Could you check a few things on this model? Use its own coordinates, in mm. Round coordinates to 2 decimals unless told otherwise and drop trailing zeros. Loops run counter-clockwise (first coordinate to the right, second up) from the corner with the lowest first, then second, coordinate; pieces in that order, holes last. Notation, with made-up numbers: (-27.5, -30.75) -> (-12.5, -30.75) arc R31 cw to (-12.5, 4.25) -> close; hole circle Ø10 at (62.5, 13.5). An arc over 180 degrees is marked (long way). Write each question's results on one line, items separated by ' | '. Start each with the question number.
1) For P1, Ø1, axis at y = -4, z = 2, coming from the -X side; P2, Ø2, axis at x = 141, z = 2, coming from the -Y side, each with a flat end and sliding along its axis, tell me the tip position at first contact or that it passes through.
2) Imagine slicing it at A-A, the plane z = 1. Give the number of separate pieces and of enclosed holes in the cut face, plus the area to 3 significant figures.
3) If I drill on probe 1 along X at (y, z) = (-7.5, 4.75); probe 2 along Y at (x, z) = (153, 2.75); probe 3 along X at (y, z) = (-2, 1.75), over which ranges is the centre line in solid material (lowest first)?
4) Imagine slicing it at C-C, the plane y = -27. List the corners of the cut face in (x, z) for me, plus the area to 3 significant figures.
5) Imagine slicing it at B-B, the plane x = 162.5. List the corners of the cut face in (y, z) for me, plus the area to 3 significant figures.
from build123d import *

# Parameters (mm, degrees)
BOSS_EXTRUDE1_DEPTH       = 6.604
F_6_CLEARANCE_HOLE1_D     = 3.6576
F_6_CLEARANCE_HOLE1_DEPTH = 10.16
F_6_CLEARANCE_HOLE1_TIP   = 1.0988539


with BuildPart() as part:
    # Sketch1 → Boss-Extrude1 (new body)
    with BuildSketch(Plane.XY):
        with BuildLine():
            Line((16.823092539, -23.059379431), (270.045750863, -45.152940848))
            Line((270.045750863, -45.152940848), (271.149626418, -32.501005867))
            Line((271.149626418, -32.501005867), (18.308001968, -10.440689482))
            add(Edge.make_bspline(
                [(6.100873241, 1.761205752), (6.243998722, 1.265414493), (6.562029623, 0.258197332), (7.239782187, -1.541714319), (8.191856686, -3.521031278), (9.459597024, -5.451591955), (10.839105985, -7.00109828), (12.345816988, -8.235279198), (14.031634784, -9.215214087), (15.656369367, -9.844087266), (17.105920915, -10.226590441), (17.911821211, -10.379141677), (18.308001968, -10.440689482)],
                knots=[0, 0, 0, 0, 0.061967329, 0.123934658, 0.247869317, 0.371803975, 0.495738633, 0.619673292, 0.74360795, 0.867542608, 0.929509938, 0.991477267, 0.991477267, 0.991477267, 0.991477267], degree=3))
            Line((6.100873241, 1.761205752), (-6.100873241, -1.761205752))
            add(Edge.make_bspline(
                [(-6.100873241, -1.761205752), (-5.89459242, -2.475769135), (-5.442695686, -3.905842246), (-4.417225036, -6.62638985), (-2.877642754, -9.827164342), (-0.591083482, -13.296598328), (3.065590072, -17.362765142), (7.603197402, -20.424150011), (12.110004519, -22.072207275), (14.454118771, -22.647767765), (15.661607343, -22.877150547), (16.252804896, -22.974574297), (16.621102903, -23.030106303), (16.751262737, -23.048877832), (16.823092539, -23.059379431)],
                knots=[0, 0, 0, 0, 0.062929816, 0.125859631, 0.251719262, 0.377578894, 0.503438525, 0.755157787, 0.881017419, 0.943947234, 0.975412142, 0.991144596, 0.999010823, 1.00687705, 1.00687705, 1.00687705, 1.00687705], degree=3))
        make_face()
    extrude(amount=BOSS_EXTRUDE1_DEPTH)

    # #6 Clearance Hole1
    with Locations(Plane.XY.offset(6.604)):
        with Locations((232.641883698, -35.515346692), (44.200873241, -19.073954498)):
            Hole(F_6_CLEARANCE_HOLE1_D / 2, depth=F_6_CLEARANCE_HOLE1_DEPTH)
            with Locations((0, 0, -(F_6_CLEARANCE_HOLE1_DEPTH + F_6_CLEARANCE_HOLE1_TIP / 2))):  # 118° drill point
                Cone(0, F_6_CLEARANCE_HOLE1_D / 2, F_6_CLEARANCE_HOLE1_TIP, mode=Mode.SUBTRACT)


solid = part.part
Checked values:
1) P1: x = -5.56 | P2: y = -33.98
2) separate pieces: 1 | enclosed holes: 2 | area: 3,530 mm^2
3) probe 1: -3.97 to 11.47 | probe 2: -34.94 to -22.19 | probe 3: -6.03 to 7.48
4) outline: (61.99, 0) -> (208.1, 0) -> (208.1, 6.6) -> (61.99, 6.6) -> close | area: 965 mm^2
5) outline: (-35.77, 0) -> (-23.02, 0) -> (-23.02, 6.6) -> (-35.77, 6.6) -> close | area: 84.2 mm^2
